from build123d import *

# Parameters (mm, degrees)
PAD_DEPTH       = 5
SKETCH001_R     = 1.7
SKETCH001_R_2   = 8.2
POCKET_DEPTH    = 5.001
SKETCH002_R     = 2.95
POCKET001_DEPTH = 3.5


with BuildPart() as part:
    # Sketch → Pad (new body)
    with BuildSketch(Plane.XY):
        with BuildLine():
            ThreePointArc((24.4, -71.131428), (75.2, 0), (24.4, 71.131428))
            Line((24.4, 71.131428), (43.268572, 90))
            Line((43.268572, 90), (219.4, 90))
            Line((219.4, 90), (219.4, -90))
            Line((219.4, -90), (43.268572, -90))
            Line((43.268572, -90), (24.4, -71.131428))
        make_face()
    extrude(amount=PAD_DEPTH)

    # Sketch001 (on Face8 of Pad) → Pocket (cut, through all)
    with BuildSketch(Plane.XY.offset(5)):
        with Locations((39.4, 75)):
            Circle(SKETCH001_R)
        with Locations((39.4, -75)):
            Circle(SKETCH001_R)
        with Locations((208.4, -80)):
            Circle(SKETCH001_R)
        with Locations((208.4, 80)):
            Circle(SKETCH001_R)
        with Locations((74.4, 67.5)):
            Circle(SKETCH001_R_2)
        with Locations((74.4, -67.5)):
            Circle(SKETCH001_R_2)
    extrude(amount=-POCKET_DEPTH, mode=Mode.SUBTRACT)

    # Sketch002 (on Face5 of Pocket) → Pocket001 (cut)
    with BuildSketch(Plane.XY.offset(5)):
        with Locations((39.4, -75)):
            Circle(SKETCH002_R)
        with Locations((208.4, -80)):
            Circle(SKETCH002_R)
        with Locations((39.4, 75)):
            Circle(SKETCH002_R)
        with Locations((208.4, 80)):
            Circle(SKETCH002_R)
    extrude(amount=-POCKET001_DEPTH, mode=Mode.SUBTRACT)


solid = part.part
Model file for the job. Use its own axes, mm. A direction names the side the tool comes from. Give positions to 0.01 mm unless a question says otherwise; leave off trailing zeros. Order: outer loops, then holes, each group sorted by start corner. A loop starts at its lowest first (then second) coordinate and runs counter-clockwise, first axis right, second up. Notation, with made-up numbers: (25.5, 32) -> (79.5, 32) arc R27 cw to (79.5, 69) -> close; hole circle Ø2 at (78, 44). An arc over 180 degrees is marked (long way). Use CSV: the item, a comma, the result in double quotes.
1. Band-saw the part on A-A, the plane z = 4.2. Give the cut face in (x, y), then the cut area to 3 significant figures.
Outcome:
outline,"(24.4, -71.13) -> (43.27, -90) -> (219.4, -90) -> (219.4, 90) -> (43.27, 90) -> (24.4, 71.13) arc R75.2 cw to start; hole circle Ø5.9 at (39.4, -75); hole circle Ø5.9 at (39.4, 75); hole circle Ø16.4 at (74.4, -67.5); hole circle Ø16.4 at (74.4, 67.5); hole circle Ø5.9 at (208.4, -80); hole circle Ø5.9 at (208.4, 80)"
area,"28,900 mm²"
2. Drop a flat-ended pin along its axis: pin 1 (4.5 mm diameter, centred on x = 208.4, y = -80, fed in from +Z). Give the stop position or say it passes through.
Outcome:
pin 1,"z = 1.5"
3. Drill centre lines: line 1 along Y through (x, z) = (208.4, 1.05); line 2 along Y through (x, z) = (208.4, 4.25); line 3 along X through (y, z) = (64.5, 1.1). Where is each one in solid material? Low to high. Write a range as from..to.
Outcome:
line 1,"-90..-81.7, -78.3..78.3, 81.7..90"
line 2,"-90..-82.95, -77.05..77.05, 82.95..90"
line 3,"38.66..66.77, 82.03..219.4"
4. Band-saw the part on B-B, the plane x = 72. Give the cut face in (y, z).
Outcome:
outline,"(-90, 0) -> (-75.34, 0) -> (-75.34, 5) -> (-90, 5) -> close; (-59.66, 0) -> (-21.7, 0) -> (-21.7, 5) -> (-59.66, 5) -> close; (21.7, 0) -> (59.66, 0) -> (59.66, 5) -> (21.7, 5) -> close; (75.34, 0) -> (90, 0) -> (90, 5) -> (75.34, 5) -> close"
5. Band-saw the part on C-C, the plane x = 49. Give the cut face in (y, z).
Outcome:
outline,"(-90, 0) -> (-57.04, 0) -> (-57.04, 5) -> (-90, 5) -> close; (57.04, 0) -> (90, 0) -> (90, 5) -> (57.04, 5) -> close"
6. 3-axis set-ups, long thin cutter, end or side, ignore diameter. For faces 5 (the cylindrical face through (211.214, 80.886, 3.274)), 6 (the flat face through (33.97, -80.7, 2.46)): which of +Z, -Z, +X, -X, +Y, -Y reach the whole face in a straight line?
Outcome:
face 5,"+Z"
face 6,"+Z, -Z, -X, -Y"
7. Mould opens along Y. For faces 1 (the flat face through (210, 79, 1.5)), 2 (the flat face through (145, 1, 5)), 3 (the flat face through (130, 90, 2)), 4 (the cylindrical face through (75.19, -1.31, 2.46)) say: +Y half, -Y half, draft (parallel to the pull), parting line (faces both ways), or undercut.
Outcome:
face 1,"undercut"
face 2,"draft"
face 3,"+Y half"
face 4,"undercut"
